Job drawing, mm, ordinate dimensions from the low corner. One solid piece. Give positions to 0.01 mm unless a question says otherwise; leave off trailing zeros. Order: outer loops, then holes, each group sorted by start corner. A loop starts at its lowest first (then second) coordinate and runs counter-clockwise, first axis right, second up.
1. Slice it at A-A on z = 86.5. Give the number of separate pieces and of enclosed holes in the cut face.
2. Probe line 1 (Z direction, x = 7.5, y = 6.25) (1 decimal); line 2 (X direction, y = 6.25, z = 86.5) (1 decimal); line 3 (Z direction, x = 96, y = 4.5). List the from-to ranges inside material, lowest first.
3. Drop flat-ended pins along their axis: pin 1 Ø1.9 at (x, y) = (138.5, 3) entering from -Z; pin 2 Ø3 at (y, z) = (4, 87.5) entering from -X; pin 3 Ø3 at (y, z) = (4.5, 24) entering from -X. Give the stop position or say it passes through.
4. Slice it at B-B on x = 17. List the corners of the cut face in (y, z), and give its area (3 significant figures).
5. Slice it at C-C on z = 23. List the corners of the cut face in (x, y).
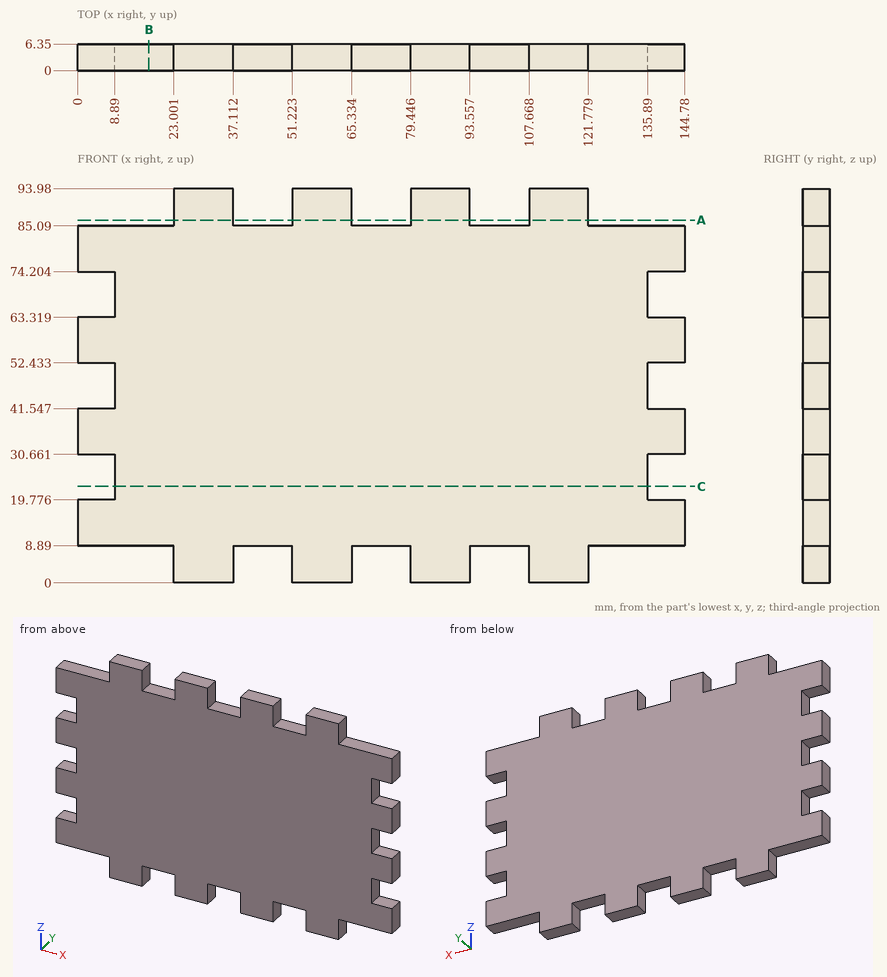
Data:
1. separate pieces: 4
1. enclosed holes: 0
2. line 1: z = 8.9 to 19.8, 30.7 to 41.5, 52.4 to 63.3, 74.2 to 85.1
2. line 2: x = 23 to 37.1, 51.2 to 65.3, 79.4 to 93.6, 107.7 to 121.8
2. line 3: z = 8.89 to 85.09
3. pin 1: stops at z = 8.89
3. pin 2: stops at x = 23
3. pin 3: stops at x = 8.89
4. outline: (0, 8.89) - (6.35, 8.89) - (6.35, 85.09) - (0, 85.09) - close
4. area: 484 mm2
5. outline: (8.89, 0) - (135.89, 0) - (135.89, 6.35) - (8.89, 6.35) - close
